Geometry: final body of the model. Coordinates: model frame, mm. Give positions to 0.01 mm unless a question says otherwise; leave off trailing zeros. Write each loop counter-clockwise with the first axis right and the second up, starting at its lowest first coordinate (ties: lowest second). Pieces come first, ordered by that corner, then holes. Notation, with made-up numbers: (-35.75, 68) -> (-24.75, 68) arc R23 ccw to (-24.75, 89) -> close; hole circle Ø3 at (-8, 77). An arc over 180 degrees is marked (long way). Answer in a Markdown table with one row per item. Add a question column.
from build123d import *

# Parameters (mm, degrees)
SKETCH1_R               = 14.25
SKETCH1_R_2             = 4
BOSS_EXTRUDE1_DEPTH     = 3.175
M4_CLEARANCE_HOLE1_D    = 4.5
VENTHOLES_DEPTH         = 65.263003169
CIRPATTERN1_COUNT       = 4
CUT_EXTRUDE2_DEPTH      = 65.263003169
SKETCH7_W               = 68.017867909
SKETCH7_H               = 13.211155311
CUT_EXTRUDE3_DEPTH      = 65.263003169
CUT_EXTRUDE3_DEPTH_BACK = 65.263003169
CUT_EXTRUDE4_DEPTH      = 52.625675669
CUT_EXTRUDE4_DEPTH_BACK = 52.625675669
CUT_EXTRUDE5_DEPTH      = 52.625675669
CUT_EXTRUDE5_DEPTH_BACK = 52.625675669
FILLET1_R               = 1


with BuildPart() as part:
    # Sketch1 → Boss-Extrude1 (new body)
    with BuildSketch(Plane.XY):
        Polygon((30.444907858, -32.62998798), (-37.572960051, -32.62998798), (-37.572960051, 52.037732697), (30.444907858, 48.473067289), align=None)
        Circle(SKETCH1_R, mode=Mode.SUBTRACT)
        with Locations((-29.572960051, -7.37834899)):
            Circle(SKETCH1_R_2, mode=Mode.SUBTRACT)
        with Locations((-11.413340062, 28.261911978)):
            Circle(SKETCH1_R_2, mode=Mode.SUBTRACT)
        with Locations((22.444907858, 11.010272988)):
            Circle(SKETCH1_R_2, mode=Mode.SUBTRACT)
        with Locations((4.285287868, -24.62998798)):
            Circle(SKETCH1_R_2, mode=Mode.SUBTRACT)
    extrude(amount=BOSS_EXTRUDE1_DEPTH)

    # M4 Clearance Hole1 (through all)
    with Locations(Plane(origin=(0, 0, 0), x_dir=(-1, 0, 0), z_dir=(0, 0, -1))):
        with Locations((-14.86289651, 13.382612127), (13.382612127, 14.86289651), (14.86289651, -13.382612127), (-13.382612127, -14.86289651)):
            Hole(M4_CLEARANCE_HOLE1_D / 2)

    # Sketch4 → VentHoles (cut, through all)
    with BuildSketch(Plane.XY):
        with BuildLine():
            ThreePointArc((-23.395136062, 29.944408637), (-30.348149382, 22.86897088), (-35.232986474, 14.23505055))
            ThreePointArc((-35.232986474, 14.23505055), (-34.127831951, 11.631469654), (-31.524251055, 12.736624176))
            ThreePointArc((-31.524251055, 12.736624176), (-27.153607342, 20.461710787), (-20.932490161, 26.792365623))
            ThreePointArc((-20.932490161, 26.792365623), (-20.587791605, 29.59971008), (-23.395136062, 29.944408637))
        make_face()
        with BuildLine():
            ThreePointArc((-18.46984426, 23.640322608), (-23.959065301, 18.054450695), (-27.815515637, 11.238197802))
            ThreePointArc((-27.815515637, 11.238197802), (-26.710361115, 8.634616906), (-24.106780219, 9.739771429))
            ThreePointArc((-24.106780219, 9.739771429), (-20.764523261, 15.647190602), (-16.007198358, 20.488279594))
            ThreePointArc((-16.007198358, 20.488279594), (-15.662499802, 23.295624052), (-18.46984426, 23.640322608))
        make_face()
        with BuildLine():
            ThreePointArc((-42.65045731, 17.231903297), (-41.545302788, 14.628322401), (-38.941721892, 15.733476923))
            ThreePointArc((-38.941721892, 15.733476923), (-33.542691422, 25.276230972), (-25.857781964, 33.096451651))
            ThreePointArc((-25.857781964, 33.096451651), (-25.513083407, 35.903796109), (-28.320427865, 36.248494666))
            ThreePointArc((-28.320427865, 36.248494666), (-36.737233462, 27.683491065), (-42.65045731, 17.231903297))
        make_face()
    ventholes = extrude(amount=VENTHOLES_DEPTH, mode=Mode.SUBTRACT)

    # CirPattern1: VentHoles ×4 about axis
    cirpattern1_axis = Axis((0, 0, 0), (0, 0, 1))
    for i in range(1, CIRPATTERN1_COUNT):
        add(ventholes.rotate(cirpattern1_axis, i * 360 / CIRPATTERN1_COUNT), mode=Mode.SUBTRACT)

    # Sketch5 → Cut-Extrude2 (cut, through all)
    with BuildSketch(Plane.XY):
        Polygon((12.341413378, 44.414969502), (11.556374035, 29.43552648), (-8.41621666, 30.482245605), (-7.631177317, 45.461688626), align=None)
    extrude(amount=CUT_EXTRUDE2_DEPTH, mode=Mode.SUBTRACT)

    # Sketch7 → Cut-Extrude3 (cut, two sides)
    with BuildSketch(Plane.XY) as cut_extrude3_sk:
        with Locations((-3.564026097, 41.867489633)):
            Rectangle(SKETCH7_W, SKETCH7_H)
    extrude(amount=CUT_EXTRUDE3_DEPTH, mode=Mode.SUBTRACT)
    extrude(cut_extrude3_sk.sketch, amount=-CUT_EXTRUDE3_DEPTH_BACK, mode=Mode.SUBTRACT)


with BuildPart() as cut_extrude3_piece_1:
    # of the separate pieces the step leaves, piece 1, a body of its own (cut_extrude3_pieces)
    add(part.part.solids().sort_by_distance((26.443976335, -32.62998798, 0))[0])

    # Sketch9 → Cut-Extrude4 (cut, two sides)
    with BuildSketch(Plane.XY.offset(3.175)) as cut_extrude4_sk:
        with BuildLine():
            ThreePointArc((24.064301101, 17.238521309), (22.71543741, 15.347484158), (20.488279594, 16.007198358))
            Line((20.488279594, 16.007198358), (20.488279594, 14.499055847))
            ThreePointArc((20.488279594, 14.499055847), (22.256357537, 15.005826613), (24.064301101, 14.667808432))
            Line((24.064301101, 14.667808432), (24.064301101, 17.238521309))
        make_face()
    extrude(amount=CUT_EXTRUDE4_DEPTH, mode=Mode.SUBTRACT)
    extrude(cut_extrude4_sk.sketch, amount=-CUT_EXTRUDE4_DEPTH_BACK, mode=Mode.SUBTRACT)

    # Sketch10 → Cut-Extrude5 (cut, two sides)
    with BuildSketch(Plane.XY.offset(3.175)) as cut_extrude5_sk:
        Polygon((-37.572960051, -32.62998798), (-30.450066979, -32.62998798), (-34.672473159, -25.089104914), (-37.572960051, -25.089104914), align=None)
        Polygon((30.444907858, 36.985955285), (11.775698683, 36.985955285), (28.36838713, 20.163813112), (30.444907858, 20.163813112), align=None)
        with BuildLine():
            Line((-37.572960051, 18.768928392), (-37.572960051, 11.485837363))
            Line((-37.572960051, 11.485837363), (-33.378618764, 11.485837363))
            ThreePointArc((-33.378618764, 11.485837363), (-35.03669391, 12.367451556), (-35.232986474, 14.23505055))
            ThreePointArc((-35.232986474, 14.23505055), (-30.348149382, 22.86897088), (-23.395136062, 29.944408637))
            ThreePointArc((-23.395136062, 29.944408637), (-21.287070818, 30.165975222), (-20.163813112, 28.36838713))
            Line((-20.163813112, 28.36838713), (-20.163813112, 35.261911978))
            Line((-20.163813112, 35.261911978), (-25.17793724, 35.261911978))
            ThreePointArc((-25.17793724, 35.261911978), (-25.180933948, 34.073404246), (-25.857781964, 33.096451651))
            ThreePointArc((-25.857781964, 33.096451651), (-32.514369728, 26.586006868), (-37.572960051, 18.768928392))
        make_face()
    extrude(amount=CUT_EXTRUDE5_DEPTH, mode=Mode.SUBTRACT)
    extrude(cut_extrude5_sk.sketch, amount=-CUT_EXTRUDE5_DEPTH_BACK, mode=Mode.SUBTRACT)

    # Fillet1
    fillet1_edges = [cut_extrude3_piece_1.edges().sort_by_distance(p)[0] for p in [
        (30.444907858, -28.932811573, 1.5875),
        (26.443976335, -32.62998798, 1.5875),
        (-11.631234454, -32.62998798, 1.5875),
        (-19.475212051, -32.62998798, 1.5875),
        (11.714368197, 32.450234687, 1.5875),
        (-8.16572496, 35.261911978, 1.5875),
        (-26.443976335, -32.62998798, 1.5875),
        (11.556374035, 29.43552648, 1.5875),
        (-8.395017915, 30.886741766, 1.5875),
        (-8.07427182, 30.464325035, 1.5875),
        (20.488279594, 16.007198358, 1.5875),
        (20.488279594, 14.499055847, 1.5875),
        (24.064301101, 14.667808432, 1.5875),
        (30.444907858, -22.739999682, 1.5875),
        (-37.572960051, -25.089104914, 1.5875),
        (30.444907858, -15.136300259, 1.5875),
        (30.444907858, 20.163813112, 1.5875),
        (-20.163813112, 35.261911978, 1.5875),
        (-37.572960051, 11.485837363, 1.5875),
    ]]
    fillet(fillet1_edges, radius=FILLET1_R)


with BuildPart() as cut_extrude3_piece_2:
    # of the separate pieces the step leaves, piece 2, a body of its own (cut_extrude3_pieces)
    add(part.part.solids().sort_by_distance((30.444907858, 48.473067289, 0))[0])


with BuildPart() as cut_extrude3_piece_3:
    # of the separate pieces the step leaves, piece 3, a body of its own (cut_extrude3_pieces)
    add(part.part.solids().sort_by_distance((-37.572960051, 35.261911978, 0))[0])


with BuildPart() as cut_extrude3_piece_4:
    # of the separate pieces the step leaves, piece 4, a body of its own (cut_extrude3_pieces)
    add(part.part.solids().sort_by_distance((29.539762417, 35.261911978, 0))[0])


with BuildPart() as cut_extrude3_piece_5:
    # of the separate pieces the step leaves, piece 5, a body of its own (cut_extrude3_pieces)
    add(part.part.solids().sort_by_distance((11.86172196, 35.261911978, 0))[0])


solid = cut_extrude3_piece_1.part
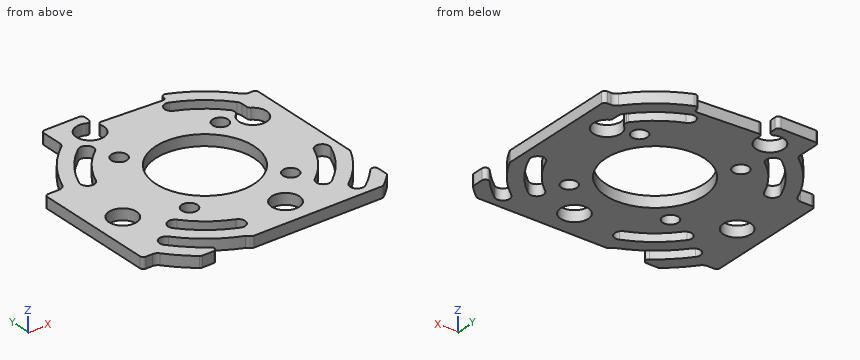
Q1. Section C-C on y = 0. Return loops of the section in (x, z) (3 decimals).
Q2. Section D-D on x = 1.5. Return loops of the section in (y, z) (3 decimals), and give its area (3 significant figures).
Q3. Contact query for flat-ended pins moving along their axis: pin 1 Ø1.6 at (y, z) = (30, 2) entering from -X; pin 2 Ø5 at (x, y) = (-11.41, 28.26) entering from -Z; pin 3 Ø3 at (x, y) = (10.5, 20.5) entering from -Z; pin 4 Ø0.6 at (x, z) = (-35.5, 1.5) entering from -Y. Output: stop coordinate, or through.
Q4. Section A-A on y = 26. Return loops of the section in (x, z) (3 decimals).
Q5. Section B-B on x = -5.5. Return loops of the section in (y, z) (3 decimals), and give its area (3 significant figures).
Q6. Line query: probe 1 along X at (y, z) = (12.5, 1.3); probe 2 along Y at (x, z) = (-9, 1.7); probe 3 along Y at (x, z) = (15, 2.45). Output: solid intervals per line, ascending. Write a range as from..to.
Checks:
| question | item | result |
|---|---|---|
| 1 | outline | (-37.573, 0) -> (-14.25, 0) -> (-14.25, 3.175) -> (-37.573, 3.175) -> close; (14.25, 0) -> (30.445, 0) -> (30.445, 3.175) -> (14.25, 3.175) -> close |
| 2 | outline | (-32.63, 0) -> (-27.501, 0) -> (-27.501, 3.175) -> (-32.63, 3.175) -> close; (-21.759, 0) -> (-14.171, 0) -> (-14.171, 3.175) -> (-21.759, 3.175) -> close; (14.171, 0) -> (29.963, 0) -> (29.963, 3.175) -> (14.171, 3.175) -> close |
| 2 | area | 90.5 mm^2 |
| 3 | pin 1 | x = -20.16 |
| 3 | pin 2 | through |
| 3 | pin 3 | z = 0 |
| 3 | pin 4 | y = -25.09 |
| 4 | outline | (-21.909, 0) -> (-14.712, 0) -> (-14.712, 3.175) -> (-21.909, 3.175) -> close; (-8.114, 0) -> (8.489, 0) -> (8.489, 3.175) -> (-8.114, 3.175) -> close; (14.967, 0) -> (21.909, 0) -> (21.909, 3.175) -> (14.967, 3.175) -> close |
| 5 | outline | (-32.63, 0) -> (-13.146, 0) -> (-13.146, 3.175) -> (-32.63, 3.175) -> close; (13.146, 0) -> (30.329, 0) -> (30.329, 3.175) -> (13.146, 3.175) -> close |
| 5 | area | 116 mm^2 |
| 6 | probe 1 | -31.64..-27.27, -22.8..-6.84, 6.84..12.79, 16.93..18.73, 26.16..30.44 |
| 6 | probe 2 | -32.63..-27.3, -24.63..-11.05, 11.05..25.07, 31.84..35.24 |
| 6 | probe 3 | -32.63..-16.43, -13.3..11.14, 15.63..21.24, 25.98..30.51 |
